For this review, take the finished solid that the model builds, in its own axes (mm). A direction names the side the tool comes from. Round coordinates to 2 decimals unless told otherwise and drop trailing zeros. Loops run counter-clockwise (first coordinate to the right, second up) from the corner with the lowest first, then second, coordinate; pieces in that order, holes last.
1) Insertion check: pin 1 (2 mm diameter, centred on x = 33.5, y = 0.5, fed in from +Z); pin 2 (1 mm diameter, centred on x = 7, z = 27.5, fed in from -Y); pin 3 (3.5 mm diameter, centred on x = 37.05, z = 29.19, fed in from +Y); pin 4 (5 mm diameter, centred on x = 11, y = -5.5, fed in from +Z). Each pin has a flat end and moves straight along its axis. Give the tip position at first contact, or say it passes through.
2) Take a section at C-C (x = 41.5). State the section outline as (y, z) points.
3) Wall thickness on L1, parallel to X at y = -1.75, z = 30.5; L2, parallel to X at y = -4.5, z = 11.5; L3, parallel to Y at x = 18, z = 10: over which ranges is each line inside the solid? List them lowest first.
4) Tool access review of faces 5 (the cylindrical face through (28.928, 0.986, -2.443)), 6 (the flat face through (43.346, 1, 13)), 7 (the flat face through (43.346, -5, 5)), 8 (the flat face through (46, 0, 13)): name each direction out of +Z, -Z, +X, -X, +Y, -Y from which nothing blocks a thin tool from reaching the whole face with its end or side.
5) Mouldability with a two-part tool opening along X and no side actions: class faces 1 (the cylindrical face through (60.58, 0.986, 32.734)), 2 (the flat face through (31, 2, 21)), 3 (the cylindrical face through (28.928, -5.435, 44.443)), 4 (the flat face through (48.296, -5, 13)) as pulls with the +X half, pulls with the -X half, needs draft (parallel to the pull), parting line crosses it, or undercut.
6) Take a section at A-A (z = 17.5). State the section outline as (x, y) points, then the cut area to 3 significant figures.
7) Take a section at B-B (y = -4.75). Give the number of separate pieces and of enclosed holes in the cut face, then the cut area to 3 significant figures.
Autodesk Inventor part; units mm, degrees
ref_plane "YZ Plane" through (0, 0, 0) normal (1, 0, 0) x (0, 1, 0)
ref_plane "XZ Plane" through (0, 0, 0) normal (0, 1, 0) x (-1, 0, 0)
ref_plane "XY Plane" through (0, 0, 0) normal (0, 0, 1) x (1, 0, 0)
sketch "Szkic1" plane through (0, 0, 0) normal (0, 1, 0) x (-1, 0, 0)
  line L0 (0, 0) -> (0, 42)
  line L1 (-28.0748, -2.4593) -> (0, 0)
  line L2 (-59.6141, 8.5234) -> (-29.7811, -2.2373)
  circle A0 centre (-54.9356, 14.8089) radius 2.0248
  circle A1 centre (-54.9355, 27.1912) radius 2.0249
  circle A2 centre (-37.047, 29.1912) radius 2.025
  line L3 (0, 42) -> (-28.0748, 44.4593)
  line L4 (-29.7811, 44.2372) -> (-59.6141, 33.4766)
  circle A3 centre (-28.4239, 40.4745) radius 4.0001
  circle A4 centre (-58.9355, 31.5953) radius 2
  line L5 (-60.9355, 31.5953) -> (-60.9355, 10.4047)
  circle A5 centre (-58.9355, 10.4047) radius 2
  circle A6 centre (-28.4239, 1.5252) radius 3.9998
  line L6 (-43.3459, 19.1078) -> (-20.7459, 19.1078)
  line L7 (-20.7459, 19.1078) -> (-20.7459, 6.5098)
  line L8 (-20.7459, 6.5098) -> (-43.3459, 6.5098)
  line L9 (-43.3459, 6.5098) -> (-43.3459, 19.1078)
  point P0 (-40, 21)
extrude "Wyciągnięcie proste1" add sketch "Szkic1" along normal blind 2
sketch "Szkic2" plane through (0, 0, 0) normal (0, -1, 0) x (1, 0, 0)
  line L0 (4.5002, 37.877) -> (28.9526, 40.019)
  line L1 (28.9526, 19.1078) -> (28.9526, 40.019)
  line L2 (43.3459, 19.1078) -> (48.2961, 19.1078)
  line L3 (48.2961, 6.5098) -> (48.2961, 19.1078)
  line L4 (43.3461, 2.6556) -> (43.3461, 6.5098)
  line L5 (48.2961, 6.5098) -> (43.3459, 6.5098)
  circle A0 centre (58.9357, 10.4048) radius 2
  line L6 (59.6143, 33.4767) -> (59.5948, 33.4837)
  circle A1 centre (58.9355, 31.5953) radius 2.0002
  line L7 (4.5002, 37.877) -> (4.5002, -0.3941)
  line L8 (28.075, -2.4592) -> (28.052, -2.4572)
  arc A2 (60.9355, 31.5953) -> (59.6141, 33.4766) centre (58.9355, 31.5953) ccw
  arc A3 (59.6141, 8.5234) -> (60.9355, 10.4047) centre (58.9355, 10.4047) ccw
  circle A4 centre (37.047, 29.1912) radius 2.025
  circle A5 centre (54.9356, 14.8089) radius 2.0248
  circle A6 centre (54.9355, 27.1912) radius 2.0249
  line L9 (0, 42) -> (28.0748, 44.4593)
  line L10 (0, 0) -> (0, 42)
  line L11 (28.0748, -2.4593) -> (0, 0)
  arc A7 (28.0748, -2.4593) -> (29.7811, -2.2372) centre (28.4239, 1.5252) ccw
  line L12 (59.6141, 8.5234) -> (29.7811, -2.2372)
  arc A8 (59.6141, 8.5234) -> (60.9355, 10.4047) centre (58.9355, 10.4047) ccw
  line L13 (60.9355, 31.5953) -> (60.9355, 10.4047)
  arc A9 (60.9355, 31.5953) -> (59.6141, 33.4766) centre (58.9355, 31.5953) ccw
  line L14 (29.7811, 44.2372) -> (59.6141, 33.4766)
  arc A10 (29.7811, 44.2372) -> (28.0748, 44.4593) centre (28.4239, 40.4745) ccw
  circle A11 centre (37.047, 29.1912) radius 2.025
  circle A12 centre (54.9356, 14.8089) radius 2.0248
  circle A13 centre (54.9355, 27.1912) radius 2.0249
  line L15 (43.3459, 6.5098) -> (43.3459, 19.1078)
  line L16 (20.7459, 6.5098) -> (43.3459, 6.5098)
  line L17 (20.7459, 19.1078) -> (20.7459, 6.5098)
  line L18 (43.3459, 19.1078) -> (20.7459, 19.1078)
  line L19 (4.5002, -0.3941) -> (4.5002, -2.2372)
  line L20 (28.9526, 19.1078) -> (28.9526, 16.8338)
  line L21 (43.3459, 6.5098) -> (42.3677, 6.5098)
  line L22 (43.3459, 6.5098) -> (43.3459, 8.4048)
  line L23 (43.3459, 6.5098) -> (43.3459, 19.1078)
  line L24 (43.3459, 19.1078) -> (42.3677, 19.1078)
  line L25 (43.3459, 19.1078) -> (43.3459, 17.9708)
  point P0 (40.0002, 21.0001)
  point P1 (59.6047, 8.52)
  point P2 (60.9355, 10.4349)
  point P3 (60.9355, 31.5648)
  point P4 (59.5854, 33.487)
  point P5 (4.5002, -0.3942)
  point P6 (28.9526, 19.1078)
  point P7 (43.3461, 2.6556)
extrude "Wyciągnięcie proste2" add sketch "Szkic2" along normal blind 11.024 contours L7 L11 L10 L9 A10 L14 A1 L13 A0 L12 L4 L5 L3 L2 L18 L1 L0 | A0 | L6 A1
sketch "Szkic3" plane through (43.3459, 2, 19.1078) normal (0, 0, -1) x (-1, 0, 0)
  circle A0 centre (35.5684, -7.5107) radius 2.1003
  point P0 (43.3459, -2)
extrude "Wyciągnięcie proste3" cut sketch "Szkic3" against normal through all
properties part number "base_edited"
Response:
1. pin 1: stops at z = 43.26
1. pin 2: stops at y = 0
1. pin 3: passes through
1. pin 4: stops at z = 43.18
2. outline: (-11.02, 19.11) - (2, 19.11) - (2, 40.01) - (-11.02, 40.01) - close; (0, 1.99) - (2, 1.99) - (2, 6.51) - (0, 6.51) - close
3. L1: x = 0 to 4.5, 28.95 to 35.5, 38.59 to 60.94
3. L2: x = 0 to 4.5, 48.3 to 60.94
3. L3: y = 0 to 2
4. face 5: -Z, +Y, -Y
4. face 6: +Y, -Y
4. face 7: -Z, -Y
4. face 8: -Y
5. face 1: pulls with the +X half
5. face 2: needs draft
5. face 3: parting line crosses it
5. face 4: undercut
6. outline: (0, -11.02) - (4.5, -11.02) - (4.5, 0) - (20.75, 0) - (20.75, 2) - (0, 2) - close; (43.35, 0) - (48.3, 0) - (48.3, -11.02) - (60.94, -11.02) - (60.94, 2) - (43.35, 2) - close
6. area: 266 mm2
7. separate pieces: 2
7. enclosed holes: 3
7. area: 1,040 mm2
